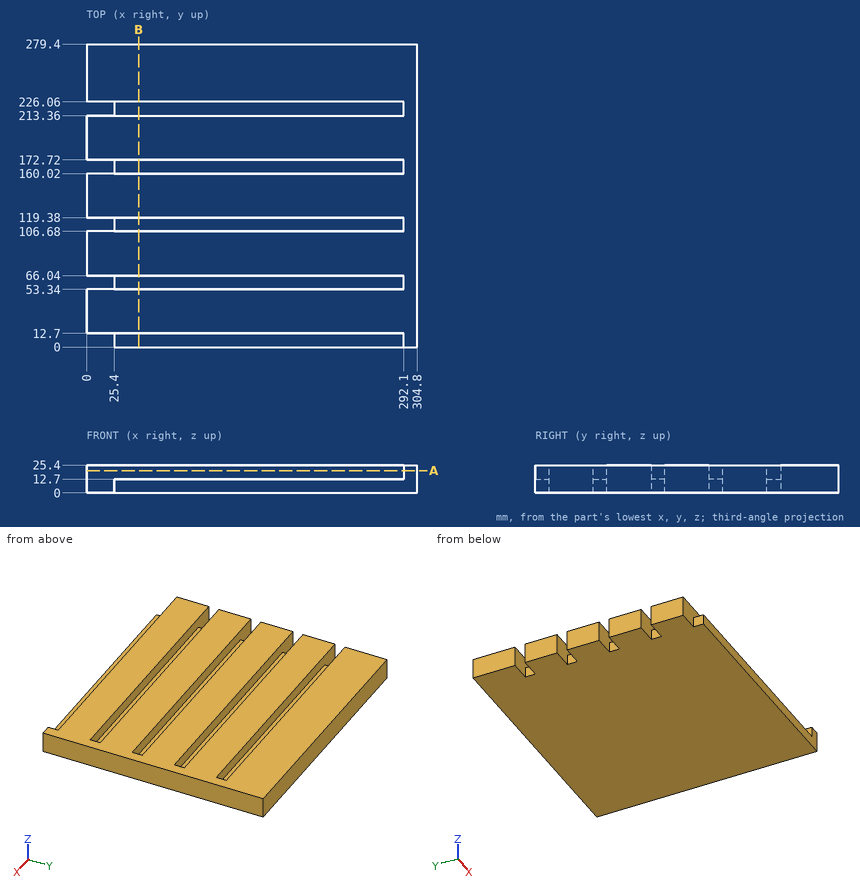
Study the drawing (mm; zero at the part's minimum x, y, z) and answer. Round coordinates to 2 decimals unless told otherwise and drop trailing zeros. Loops run counter-clockwise (first coordinate to the right, second up) from the corner with the lowest first, then second, coordinate; pieces in that order, holes last.
Q1. Given pin 1 Ø5 at (y, z) = (166.5, 8.5) entering from -X; pin 2 Ø4 at (x, y) = (197.5, 221) entering from +Z; pin 3 Ø4 at (y, z) = (60, 19) entering from -X, each flat-ended and moving along its own axis, determine where each tip first touches the part or whether it passes through.
Q2. Section B-B, the plane x = 48 is taken. Determine the outline of the cut face in (y, z).
Q3. Section A-A, the plane z = 20.5 is taken. Determine the outline of the cut face in (x, y), then the cut area to 3 significant figures.
Q4. Find the intervals of material crossed by line 1 (Y direction, x = 161, z = 13); line 2 (X direction, y = 169, z = 22.25), in increasing order.
Completed:
1. pin 1: stops at x = 25.4
1. pin 2: stops at z = 12.7
1. pin 3: stops at x = 292.1
2. outline: (0, 0) - (279.4, 0) - (279.4, 25.4) - (226.06, 25.4) - (226.06, 12.7) - (213.36, 12.7) - (213.36, 25.4) - (172.72, 25.4) - (172.72, 12.7) - (160.02, 12.7) - (160.02, 25.4) - (119.38, 25.4) - (119.38, 12.7) - (106.68, 12.7) - (106.68, 25.4) - (66.04, 25.4) - (66.04, 12.7) - (53.34, 12.7) - (53.34, 25.4) - (12.7, 25.4) - (12.7, 12.7) - (0, 12.7) - close
3. outline: (0, 12.7) - (292.1, 12.7) - (292.1, 0) - (304.8, 0) - (304.8, 279.4) - (0, 279.4) - (0, 226.06) - (292.1, 226.06) - (292.1, 213.36) - (0, 213.36) - (0, 172.72) - (292.1, 172.72) - (292.1, 160.02) - (0, 160.02) - (0, 119.38) - (292.1, 119.38) - (292.1, 106.68) - (0, 106.68) - (0, 66.04) - (292.1, 66.04) - (292.1, 53.34) - (0, 53.34) - close
3. area: 66,600 mm2
4. line 1: y = 12.7 to 53.34, 66.04 to 106.68, 119.38 to 160.02, 172.72 to 213.36, 226.06 to 279.4
4. line 2: x = 292.1 to 304.8
